Verification items for the finished model (mm, model axes). A direction names the side the tool comes from. Give positions to 0.01 mm unless a question says otherwise; leave off trailing zeros. Write each loop counter-clockwise with the first axis right and the second up, starting at its lowest first coordinate (ties: lowest second). Pieces come first, ordered by that corner, then holes.
from build123d import *

# Parameters (mm, degrees)
SKETCH1_W           = 150
SKETCH1_H           = 200
PLATE_DEPTH         = 19.05
SKETCH2_W           = 150
SKETCH2_H           = 19.05
BOSS_EXTRUDE1_DEPTH = 150
BOSS_EXTRUDE2_DEPTH = 19.05
SKETCH4_R           = 3.175
CUT_EXTRUDE1_DEPTH  = 292.547594742
SKETCH6_R           = 3
CUT_EXTRUDE2_DEPTH  = 290.518229132


with BuildPart() as part:
    # Sketch1 → Plate (new body)
    with BuildSketch(Plane.XY):
        with Locations((75, 100)):
            Rectangle(SKETCH1_W, SKETCH1_H)
    extrude(amount=PLATE_DEPTH)

    # Sketch2 → Boss-Extrude1 (add)
    with BuildSketch(Plane.XY.offset(19.05)):
        with Locations((75, 190.475)):
            Rectangle(SKETCH2_W, SKETCH2_H)
    extrude(amount=BOSS_EXTRUDE1_DEPTH)

    # Sketch3 → Boss-Extrude2 (add)
    with BuildSketch(Plane.ZY):
        Polygon((0, 200), (0, 100), (100, 200), align=None)
    boss_extrude2 = extrude(amount=-BOSS_EXTRUDE2_DEPTH)

    # Mirror1: Boss-Extrude2 across plane
    add(boss_extrude2.mirror(Plane.ZY.offset(-75)))

    # Sketch4 → Cut-Extrude1 (cut, symmetric)
    with BuildSketch(Plane.XY.offset(19.05)):
        with Locations((61.25, 171.25)):
            Circle(SKETCH4_R)
        with Locations((61.25, 142.5)):
            Circle(SKETCH4_R)
        with Locations((61.25, 113.75)):
            Circle(SKETCH4_R)
    cut_extrude1 = extrude(amount=CUT_EXTRUDE1_DEPTH, both=True, mode=Mode.SUBTRACT)

    # Mirror2: Cut-Extrude1 across plane
    add(cut_extrude1.mirror(Plane.ZY.offset(-75)), mode=Mode.SUBTRACT)

    # Sketch6 → Cut-Extrude2 (cut, through all)
    with BuildSketch(Plane.XZ.offset(-180.95)):
        with Locations(Location((67.5, 98.5, 0), (0, 0, 270))):
            Circle(SKETCH6_R)
        with Locations(Location((82.5, 98.5, 0), (0, 0, 270))):
            Circle(SKETCH6_R)
    extrude(amount=-CUT_EXTRUDE2_DEPTH, mode=Mode.SUBTRACT)


solid = part.part
Item 1: Depth check by flat-ended pin: pin 1 (5 mm diameter, centred on x = 88.75, y = 171.25, fed in from +Z); pin 2 (1 mm diameter, centred on x = 82.5, z = 127, fed in from -Y); pin 3 (12 mm diameter, centred on x = 43, y = 159, fed in from +Z). Enter the tip coordinate at first touch or a pass-through.
Answer key:
pin 1: passes through
pin 2: stops at y = 180.95
pin 3: stops at z = 19.05
Item 2: Set-up check for faces 5 (the face through (130.95, 157, 43)), 6 (the face through (74, 200, 83)): record each of +Z, -Z, +X, -X, +Y, -Y from which the full face is reachable in a straight line by a thin tool's end or side.
Answer key:
face 5: +Z, -Y
face 6: +Z, -Z, +X, -X, +Y
Item 3: Scan lines: line 1 along Y through (x, z) = (61, 7); line 2 along X through (y, z) = (194, 98); line 3 along X through (y, z) = (142.5, 7.75) (3 decimals). Record each from-to range of solid material in increasing order.
Answer key:
line 1: y = 0 to 110.58, 116.92 to 139.33, 145.67 to 168.08, 174.42 to 200
line 2: x = 0 to 64.54, 70.46 to 79.54, 85.46 to 150
line 3: x = 0 to 58.075, 64.425 to 85.575, 91.925 to 150
Item 4: Release check for a two-part mould opening along Y. For faces 1 (the face through (80.7, 190.3, 100.9)), 2 (the face through (63, 116.4, 9.7)), 3 (the face through (85.72, 172.2, 9.66)), 4 (the face through (9, 150, 50)) record: released by +Y, released by -Y, zero draft, split by the parting line, or undercut.
Answer key:
face 1: zero draft
face 2: undercut
face 3: undercut
face 4: released by -Y
Item 5: Sectioned sample at B-B on x = 61.25. Record the cut outline in (y, z) (3 decimals), then the cut area to 3 significant figures.
Answer key:
outline: (0, 0) - (110.575, 0) - (110.575, 19.05) - (0, 19.05) - close; (116.925, 0) - (139.325, 0) - (139.325, 19.05) - (116.925, 19.05) - close; (145.675, 0) - (168.075, 0) - (168.075, 19.05) - (145.675, 19.05) - close; (174.425, 0) - (200, 0) - (200, 169.05) - (180.95, 169.05) - (180.95, 19.05) - (174.425, 19.05) - close
area: 6,300 mm2
Item 6: Sectioned sample at C-C on z = 98.5. Record the cut outline in (x, y).
Answer key:
outline: (0, 180.95) - (64.5, 180.95) - (64.5, 200) - (0, 200) - close; (70.5, 180.95) - (79.5, 180.95) - (79.5, 200) - (70.5, 200) - close; (85.5, 180.95) - (150, 180.95) - (150, 200) - (85.5, 200) - close
Item 7: Sectioned sample at A-A on y = 113.75. Record the cut outline in (x, z) (3 decimals).
Answer key:
outline: (0, 0) - (58.075, 0) - (58.075, 19.05) - (0, 19.05) - close; (64.425, 0) - (85.575, 0) - (85.575, 19.05) - (64.425, 19.05) - close; (91.925, 0) - (150, 0) - (150, 19.05) - (91.925, 19.05) - close
Item 8: Sectioned sample at D-D on x = 12. Record the cut outline in (y, z).
Answer key:
outline: (0, 0) - (200, 0) - (200, 169.05) - (180.95, 169.05) - (180.95, 80.95) - (119.05, 19.05) - (0, 19.05) - close
